from build123d import *

# Parameters (mm, degrees)
SKETCH_W     = 12.3
SKETCH_H     = 12.3
PAD_DEPTH    = 7
FILLET_R     = 3.5
CHAMFER_SIZE = 0.5
SKETCH002_R  = 4.5
PAD002_DEPTH = 0.3


with BuildPart() as part:
    # Sketch → Pad (new body)
    with BuildSketch(Plane.XY.offset(0.5)):
        Rectangle(SKETCH_W, SKETCH_H)
    extrude(amount=PAD_DEPTH)

    # Fillet
    fillet_edges = [part.edges().sort_by_distance(p)[0] for p in [
        (6.15, 6.15, 4),
        (6.15, -6.15, 4),
        (-6.15, 6.15, 4),
        (-6.15, -6.15, 4),
    ]]
    fillet(fillet_edges, radius=FILLET_R)

    # Chamfer
    chamfer_edges = [part.edges().sort_by_distance(p)[0] for p in [
        (0, 6.15, 7.5),
        (-5.124874, 5.124874, 7.5),
        (5.124874, 5.124874, 7.5),
        (-6.15, 0, 7.5),
        (6.15, 0, 7.5),
        (-5.124874, -5.124874, 7.5),
        (5.124874, -5.124874, 7.5),
        (0, -6.15, 7.5),
        (0, 6.15, 0.5),
        (-5.124874, 5.124874, 0.5),
        (5.124874, 5.124874, 0.5),
        (-6.15, 0, 0.5),
        (6.15, 0, 0.5),
        (-5.124874, -5.124874, 0.5),
        (5.124874, -5.124874, 0.5),
        (0, -6.15, 0.5),
    ]]
    chamfer(chamfer_edges, length=CHAMFER_SIZE)

    # Sketch002 (on Face11 of Chamfer) → Pad002 (join)
    with BuildSketch(Plane.XY.offset(7.5)):
        Circle(SKETCH002_R)
    extrude(amount=PAD002_DEPTH)


solid = part.part
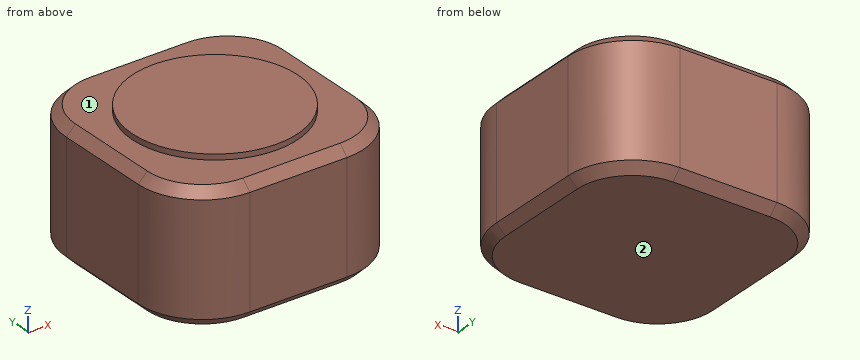
Here's how the part is built. I have some questions about the finished solid (model axes, mm). Face numbers are marked on the shaded views. A direction names the side the tool comes from. Round coordinates to 2 decimals unless told otherwise and drop trailing zeros. Write each loop counter-clockwise with the first axis right and the second up, starting at its lowest first coordinate (ties: lowest second). Pieces come first, ordered by that corner, then holes.
1. I need wall thicknesses on L1, parallel to Z at x = 5, y = 0.75; L2, parallel to Y at x = -2.75, z = 3.5; L3, parallel to Y at x = 4, z = 4.75. Which ranges of each line are inside material? Lowest first, please.
2. For the marked faces 1 and 2, which set-ups out of +Z, -Z, +X, -X, +Y, -Y let a thin tool reach every point of the face, with its end or its side?
3. Suppose I cut it at A-A (x = 0). List the corners of the cut face in (y, z) for me.
4. Suppose I cut it at C-C (z = 6.5). List the corners of the cut face in (x, y) for me.
Answer sheet:
1. L1: z = 0.5 to 7.5
1. L2: y = -6.15 to 6.15
1. L3: y = -5.88 to 5.88
2. face 1: +Z
2. face 2: -Z, +X, -X, +Y, -Y
3. outline: (-6.15, 1) - (-5.65, 0.5) - (5.65, 0.5) - (6.15, 1) - (6.15, 7) - (5.65, 7.5) - (4.5, 7.5) - (4.5, 7.8) - (-4.5, 7.8) - (-4.5, 7.5) - (-5.65, 7.5) - (-6.15, 7) - close
4. outline: (-6.15, -2.65) arc R3.5 ccw to (-2.65, -6.15) - (2.65, -6.15) arc R3.5 ccw to (6.15, -2.65) - (6.15, 2.65) arc R3.5 ccw to (2.65, 6.15) - (-2.65, 6.15) arc R3.5 ccw to (-6.15, 2.65) - close
